Work out the finished part from the listing and answer in its coordinate system (mm). A direction names the side the tool comes from. Give positions to 0.01 mm unless a question says otherwise; leave off trailing zeros. Order: outer loops, then holes, each group sorted by start corner. A loop starts at its lowest first (then second) coordinate and runs counter-clockwise, first axis right, second up.
```python
from build123d import *

# Parameters (mm, degrees)
F0_R            = 8.89
F1_DEPTH        = 12.7
F2_R            = 6.35
F3_DEPTH        = 27.94
F4_R            = 5.334
F5_DEPTH        = 40.64
F7_DEPTH        = 40.64
F7_COPIES_COUNT = 6
F8_R            = 0.508
F9_R            = 4
F10_DEPTH       = 33.02
F14_D           = 2.2606
F14_DEPTH       = 8.89
F14_START       = 0.0721476
F14_TIP         = 0.6791527577


# Not quite as in the source:
# - a pattern or mirror of a feature is missing from the dataset's text; its kind, count and spacing are read off the source's solid


with BuildPart() as f1:
    # F0 (on Top) → F1 (new body)
    with BuildSketch(Plane.XY):
        Circle(F0_R)
    extrude(amount=F1_DEPTH)

    # F2 (on face) → F3 (join)
    with BuildSketch(Plane.XY.offset(12.7)):
        Circle(F2_R)
    extrude(amount=F3_DEPTH)

    # F4 (on face) → F5 (join)
    with BuildSketch(Plane.XY.offset(40.64)):
        Circle(F4_R)
    extrude(amount=F5_DEPTH)

    # F6 (on face) → F7 (join, through all)
    with BuildSketch(Plane.XY.offset(81.28)):
        with BuildLine():
            Line((-1.27, -5.1806038258), (-1.27, -6.1957780109))
            ThreePointArc((-1.27, -6.1957780109), (0, -6.3246), (1.27, -6.1957780109))
            Line((1.27, -6.1957780109), (1.27, -5.1806038258))
            ThreePointArc((1.27, -5.1806038258), (0, -5.334), (-1.27, -5.1806038258))
        make_face()
    f7 = extrude(amount=-F7_DEPTH)

    # F7_copies: F7 ×6 about axis
    f7_copies_axis = Axis((0, 0, 0), (0, 0, 1))
    for i in range(1, F7_COPIES_COUNT):
        add(f7.rotate(f7_copies_axis, i * 360 / F7_COPIES_COUNT))

    # F8
    f8_edges = [f1.edges().sort_by_distance(p)[0] for p in [
        (1.27, -6.195778, 60.96),
        (1.27, -5.180604, 60.96),
        (-1.27, -6.195778, 60.96),
        (-1.27, -5.180604, 60.96),
        (3.851535, -3.690154, 60.96),
        (4.730701, -4.197741, 60.96),
        (6.000701, -1.998037, 60.96),
        (5.121535, -1.49045, 60.96),
        (5.121535, 1.49045, 60.96),
        (6.000701, 1.998037, 60.96),
        (4.730701, 4.197741, 60.96),
        (3.851535, 3.690154, 60.96),
        (1.27, 5.180604, 60.96),
        (1.27, 6.195778, 60.96),
        (-1.27, 6.195778, 60.96),
        (-1.27, 5.180604, 60.96),
        (-3.851535, 3.690154, 60.96),
        (-4.730701, 4.197741, 60.96),
        (-6.000701, 1.998037, 60.96),
        (-5.121535, 1.49045, 60.96),
        (-5.121535, -1.49045, 60.96),
        (-6.000701, -1.998037, 60.96),
        (-4.730701, -4.197741, 60.96),
        (-3.851535, -3.690154, 60.96),
    ]]
    fillet(f8_edges, radius=F8_R)

    # F9 (on face) → F10 (cut)
    with BuildSketch(Plane(origin=(0, 0, 0), x_dir=(1, 0, 0), z_dir=(0, 0, -1))):
        Circle(F9_R)
    extrude(amount=-F10_DEPTH, mode=Mode.SUBTRACT)

    # F14
    # its depths count from where the whole tool has entered the part; down to there all is cleared
    with Locations(Plane(origin=(-8.89, 0, 0), x_dir=(0, 1, 0), z_dir=(-1, 0, 0)).offset(-F14_START)):
        with Locations((0, -7.62)):
            Hole(F14_D / 2, depth=F14_DEPTH)
            with Locations((0, 0, -(F14_DEPTH + F14_TIP / 2))):  # 118° drill point
                Cone(0, F14_D / 2, F14_TIP, mode=Mode.SUBTRACT)


solid = f1.part
```
1. The part is cut by section B-B (x = -2.5). Write down the section's boundary in (y, z).
Findings below:
outline: (-8.53, 0) - (-3.12, 0) - (-3.12, 33.02) - (3.12, 33.02) - (3.12, 0) - (8.53, 0) - (8.53, 12.7) - (5.84, 12.7) - (5.84, 40.64) - (4.71, 40.64) - (4.71, 81.28) - (-4.71, 81.28) - (-4.71, 40.64) - (-5.84, 40.64) - (-5.84, 12.7) - (-8.53, 12.7) - close
2. The part is cut by section A-A (y = 0). Write down the section's boundary in (x, z), then the cut area to 3 significant figures.
Findings below:
outline: (-8.89, 0) - (-4, 0) - (-4, 6.49) - (-8.89, 6.49) - close; (-8.89, 8.75) - (-4, 8.75) - (-4, 33.02) - (4, 33.02) - (4, 0) - (8.89, 0) - (8.89, 12.7) - (6.35, 12.7) - (6.35, 40.64) - (5.33, 40.64) - (5.33, 81.28) - (-5.33, 81.28) - (-5.33, 40.64) - (-6.35, 40.64) - (-6.35, 12.7) - (-8.89, 12.7) - close
area: 739 mm2
3. The part is cut by section C-C (z = 7.62). Write down the section's boundary in (x, y).
Findings below:
outline: (-8.82, -1.13) arc R8.89 ccw (long way) to (-8.82, 1.13) - (-3.84, 1.13) arc R4 cw (long way) to (-3.84, -1.13) - close
4. The mould has two halves that part along Z. Classify faces 4 (the face through (2, -4, 0)), 5 (the face through (5.483, 3.152, 61.244)), 6 (the face through (4, -6, 12.7)), 7 (the face through (-6.329, -0.522, 8.623)): pulls with the +Z half, pulls with the -Z half, needs draft (parallel to the pull), parting line crosses it, or undercut.
Findings below:
face 4: pulls with the -Z half
face 5: needs draft
face 6: pulls with the +Z half
face 7: undercut
5. Which of the six approach directions +Z, -Z, +X, -X, +Y, -Y give full straight-line access (tool end or side, diameter ignored) to faces 1 (the face through (3, -5, 40.64)), 2 (the face through (5.334, -0.016, 60.676)), 3 (the face through (-5.483, -3.152, 61.244))?
Findings below:
face 1: +Z
face 2: +Z, +X
face 3: +Z, -X, -Y
6. Straight lines are drawn through the part: probe 1 along Y at (x, z) = (-7.3, 7.62); probe 2 along Y at (x, z) = (0, 25); probe 3 along Z at (x, y) = (-5.45, 0). For each, find the intervals that lie inside material, in ascending order.
Findings below:
probe 1: y = -5.07 to -1.13, 1.13 to 5.07
probe 2: y = -6.35 to -4, 4 to 6.35
probe 3: z = 0 to 6.49, 8.75 to 40.64
7. Given P1, Ø2, axis at x = 2.5, z = 24, coming from the +Y side; P2, Ø5, axis at x = -0.5, z = 23.5, coming from the +Y side; P3, Ø5, axis at y = -7, z = 43, coming from the +X side; P4, Ø10.5, axis at x = 0, y = 0, coming from the -Z side, each flat-ended and moving along its own axis, determine where each tip first touches the part or whether it passes through.
Findings below:
P1: stops at y = 6.17
P2: stops at y = 6.35
P3: stops at x = 2.86
P4: stops at z = 0
8. The part is cut by section D-D (y = -7.5). Write down the section's boundary in (x, z), then the cut area to 3 significant figures.
Findings below:
outline: (-4.77, 0) - (4.77, 0) - (4.77, 12.7) - (-4.77, 12.7) - close
area: 121 mm2
